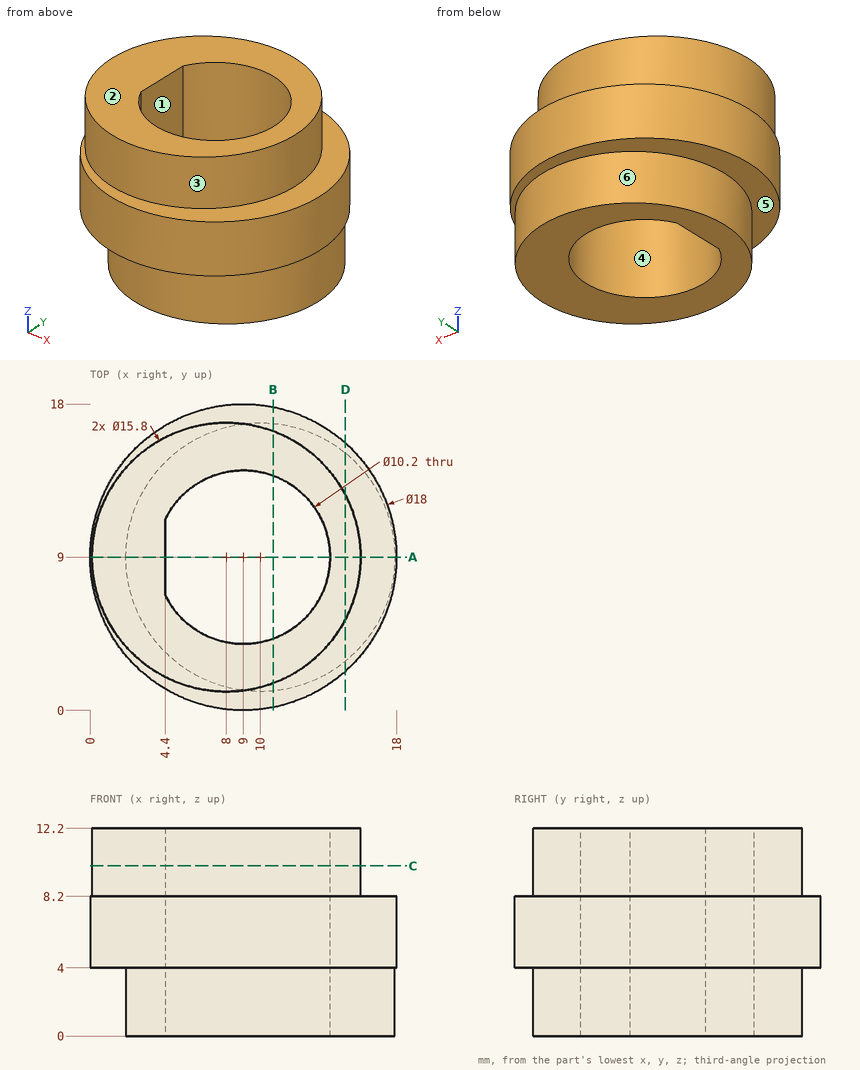
The drawing under review shows one solid part. Ordinate dimensions are in mm from its lowest x, y, z. A direction names the side the tool comes from. Round coordinates to 2 decimals unless told otherwise and drop trailing zeros. Loops run counter-clockwise (first coordinate to the right, second up) from the corner with the lowest first, then second, coordinate; pieces in that order, holes last. Notation, with made-up numbers: (-8.75, 86.5) - (1.25, 86.5) arc R10 ccw to (1.25, 91.5) - close; hole circle Ø3 at (44, -30.5). An arc over 180 degrees is marked (long way). One line per item, written item: value. Start each with the question number.
1) Insertion check: pin 1 Ø2 at (x, y) = (5.5, 10) entering from +Z; pin 2 Ø4 at (y, z) = (12, 7) entering from -X; pin 3 Ø6 at (x, y) = (6, 15.5) entering from -Z; pin 4 Ø1 at (x, z) = (2, 4.5) entering from +Y (3 decimals). Each pin has a flat end and moves straight along its axis. Give the tip position at first contact, or say it passes through.
2) Consider section C-C on z = 10. Give the boundary of the cut face in (x, y).
3) Draft analysis for pull direction X (two halves, no side actions). For the marked faces 4, 5 and 6, state which applies: +X half, -X half, draft (parallel to the pull), parting line (faces both ways), or undercut.
4) For the marked faces 1, 2 and 3, list the 3-axis set-ups (+Z, -Z, +X, -X, +Y, -Y) from which the entire face can be reached by the end or side of a thin tool; tool diameter is ignored.
5) Consider section D-D on x = 15. Give the boundary of the cut face in (y, z), then the cut area to 3 significant figures.
6) Consider section A-A on y = 9. Give the boundary of the cut face in (x, z).
7) To check wall thickness, follow L1, parallel to Y at x = 9, z = 6.75; L2, parallel to X at y = 6.75, z = 0.5; L3, parallel to X at y = 10, z = 4.75. State the ranges of each line that lie inside material, in increasing order. Write a range as from..to.
8) Consider section B-B on x = 10.75. Give the boundary of the cut face in (y, z).
Reported:
1. pin 1: passes through
1. pin 2: stops at x = 0.06
1. pin 3: stops at z = 0
1. pin 4: stops at y = 15.225
2. outline: circle Ø15.8 at (8, 9); hole (4.4, 6.8) arc R5.1 ccw (long way) to (4.4, 11.2) - close
3. face 4: undercut
3. face 5: draft
3. face 6: parting line
4. face 1: +Z, -Z
4. face 2: +Z, +X, -X, +Y, -Y
4. face 3: +Z
5. outline: (2.29, 4) - (2.88, 4) - (2.88, 0) - (15.12, 0) - (15.12, 4) - (15.71, 4) - (15.71, 8.2) - (12.66, 8.2) - (12.66, 12.2) - (5.34, 12.2) - (5.34, 8.2) - (2.29, 8.2) - close
5. area: 135 mm^2
6. outline: (0, 4) - (2.1, 4) - (2.1, 0) - (4.4, 0) - (4.4, 12.2) - (0.1, 12.2) - (0.1, 8.2) - (0, 8.2) - close; (14.1, 0) - (17.9, 0) - (17.9, 4) - (18, 4) - (18, 8.2) - (15.9, 8.2) - (15.9, 12.2) - (14.1, 12.2) - close
7. L1: y = 0..3.9, 14.1..18
7. L2: x = 2.43..4.42, 13.58..17.57
7. L3: x = 0.06..4.4, 14..17.94
8. outline: (0.17, 4) - (1.14, 4) - (1.14, 0) - (4.21, 0) - (4.21, 12.2) - (1.59, 12.2) - (1.59, 8.2) - (0.17, 8.2) - close; (13.79, 0) - (16.86, 0) - (16.86, 4) - (17.83, 4) - (17.83, 8.2) - (16.41, 8.2) - (16.41, 12.2) - (13.79, 12.2) - close
